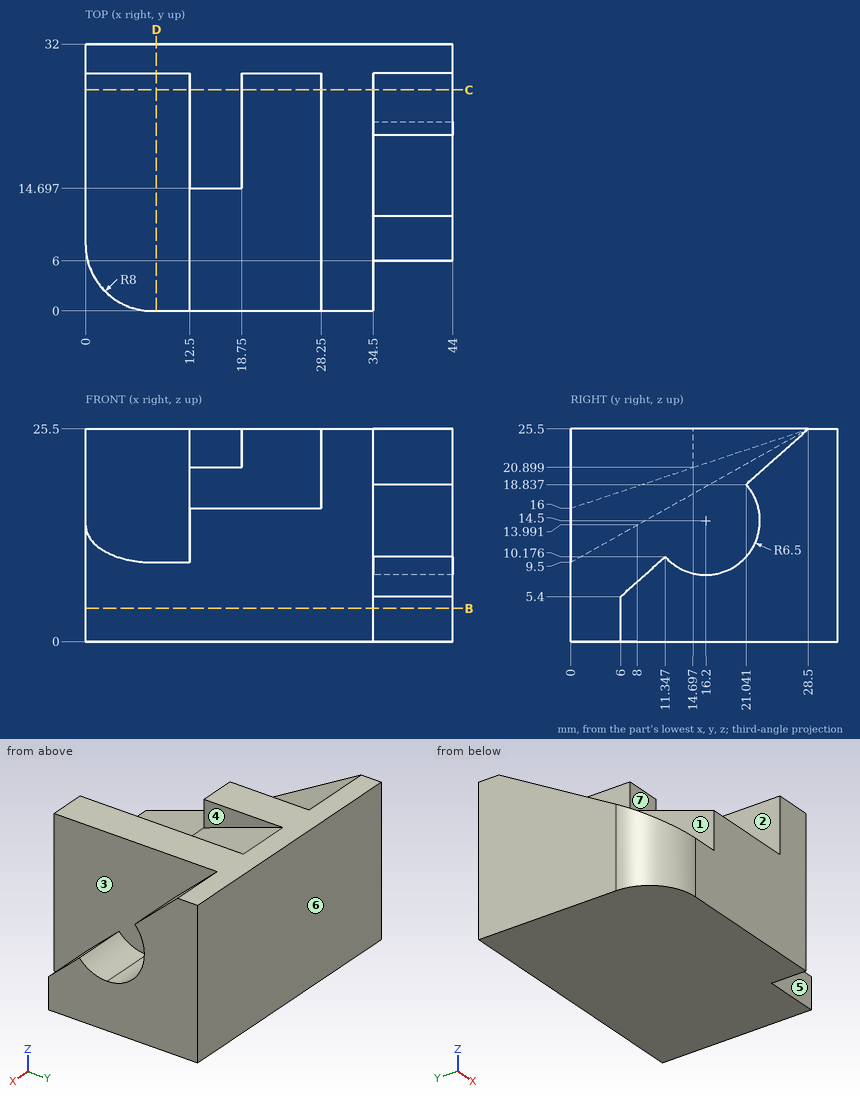
The drawing under review shows one solid part. Ordinate dimensions are in mm from its lowest x, y, z. A direction names the side the tool comes from. Give positions to 0.01 mm unless a question says otherwise; leave off trailing zeros. Order: outer loops, then holes, each group sorted by start corner. A loop starts at its lowest first (then second) coordinate and runs counter-clockwise, first axis right, second up. Notation, with made-up numbers: M 25,-39.5 L 61,-39.5 A19 ccw 61,-14.5 Z; hole C 18,11.25 d9. An arc over 180 degrees is marked long. Answer in a Markdown table with one row per item. Add a question column.
1. To check wall thickness, follow line 1 along X through (y, z) = (18.5, 22.5); line 2 along X through (y, z) = (15.5, 12.75); line 3 along X through (y, z) = (7, 18.75). State the ranges of each line that lie inside material, in increasing order.
2. Machinability: for the marked faces 4, 5, 6 and 7, which of the approach directions +Z, -Z, +X, -X, +Y, -Y give a long, thin tool a straight path to every point of the face, cutting with its end or side? Answer none if there is none.
3. Add section C-C on y = 26.5. State the section outline as (x, z) points.
4. Add section D-D on x = 8.5. State the section outline as (y, z) points, plus the area to 3 significant figures.
5. For pin 1 Ø12 at (x, z) = (11, 20) entering from -Y; pin 2 Ø2.5 at (x, z) = (37, 3.5) entering from -Y; pin 3 Ø1.4 at (x, z) = (16, 24) entering from -Y, all flat-tipped, find the tip position at first contact; note any pin that passes through.
6. Add section B-B on z = 4. State the section outline as (x, y) points, plus the area to 3 significant figures.
7. Mouldability with a two-part tool opening along X and no side actions: class the marked faces 1, 2 and 3 as released by +X, released by -X, zero draft, split by the parting line, or undercut.
The answers:
| question | item | result |
|---|---|---|
| 1 | line 1 | 12.5 to 18.75, 28.25 to 34.5 |
| 1 | line 2 | 0 to 34.5 |
| 1 | line 3 | 28.25 to 34.5 |
| 2 | face 4 | +Z, -Y |
| 2 | face 5 | +Z, -Z, +X, -Y |
| 2 | face 6 | +Z, -Z, +X, -X, +Y |
| 2 | face 7 | +Z, -X, -Y |
| 3 | outline | M 0,0 L 44,0 L 44,23.71 L 34.5,23.71 L 34.5,25.5 L 28.25,25.5 L 28.25,24.83 L 18.75,24.83 L 18.75,25.5 L 12.5,25.5 L 12.5,24.38 L 0,24.38 Z |
| 4 | outline | M 0,0 L 32,0 L 32,25.5 L 28.5,25.5 L 0,9.5 Z |
| 4 | area | 588 mm2 |
| 5 | pin 1 | y = 0 |
| 5 | pin 2 | y = 6 |
| 5 | pin 3 | y = 14.7 |
| 6 | outline | M 0,8 A8 ccw 8,0 L 34.5,0 L 34.5,6 L 44,6 L 44,32 L 0,32 Z |
| 6 | area | 1,340 mm2 |
| 7 | face 1 | released by -X |
| 7 | face 2 | undercut |
| 7 | face 3 | released by +X |
